Model file for the job. Use its own axes, mm. Face numbers are marked on the shaded views. A direction names the side the tool comes from. Coordinates: 2 decimals unless noted, no trailing zeros. Order: outer loops, then holes, each group sorted by start corner. A loop starts at its lowest first (then second) coordinate and runs counter-clockwise, first axis right, second up. Notation, with made-up numbers: M 38.25,51.25 L 43.25,51.25 A18 cw 43.25,64.25 Z; hole C 81,-14.75 d7. An arc over 180 degrees is marked long. Return JSON: item names as keys, results as strings.
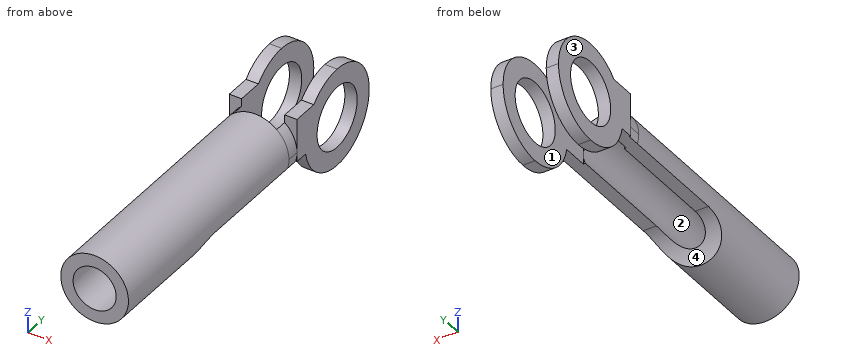
```python
from build123d import *
from build123d.topology import SkipClean

# Parameters (mm, degrees)
SKETCH_1_R               = 2.75
SKETCH_1_R_2             = 1.75
EXTRUDE_1_DEPTH          = 20
CUT_EXTRUDE_2_DEPTH      = 21.374616561
CUT_EXTRUDE_2_DEPTH_BACK = 21.374616561
SKETCH_3_W               = 1
SKETCH_3_H               = 8
EXTRUDE_3_DEPTH          = 10
SKETCH_4_R               = 2.5
CUT_EXTRUDE_5_DEPTH      = 31.761176848
CUT_EXTRUDE_8_DEPTH      = 1


with BuildPart() as part:
    # 草圖1 → 伸長1 (new body)
    with BuildSketch(Plane(origin=(0, 0, 0), x_dir=(1, 0, 0), z_dir=(0, 1, 0))):
        with Locations(Location((0, 0, 0), (0, 0, 270))):
            Circle(SKETCH_1_R)
        with Locations(Location((0, 0, 0), (0, 0, 270))):
            Circle(SKETCH_1_R_2, mode=Mode.SUBTRACT)
    extrude(amount=EXTRUDE_1_DEPTH)

    # 草圖2 → 伸長2 (cut, two sides: drawn at the far end of the back side and taken through both)
    with BuildSketch(Plane(origin=(0, 0, 0), x_dir=(0, 0, -1), z_dir=(1, 0, 0)).offset(-CUT_EXTRUDE_2_DEPTH_BACK)):
        with BuildLine():
            Line((0.75, 20), (0.75, 11.16227766))
            ThreePointArc((0.75, 11.16227766), (1.291960108, 9.291448967), (2.75, 8))
            Line((2.75, 8), (2.75, 20))
            Line((2.75, 20), (0.75, 20))
        make_face()
    extrude(amount=CUT_EXTRUDE_2_DEPTH + CUT_EXTRUDE_2_DEPTH_BACK, mode=Mode.SUBTRACT)

    # 草圖3 → 伸長3 (add)
    with BuildSketch(Plane(origin=(0, 20, 0), x_dir=(1, 0, 0), z_dir=(0, 1, 0))):
        with Locations((-2.25, 0)):
            Rectangle(SKETCH_3_W, SKETCH_3_H)
        with Locations((2.25, 0)):
            Rectangle(SKETCH_3_W, SKETCH_3_H)
    extrude(amount=EXTRUDE_3_DEPTH)

    # 草圖4 → 伸長5 (cut, through all)
    with BuildSketch(Plane.ZY.offset(2.75)):
        with BuildLine():
            Line((-4, 20), (-0.75, 20))
            Line((-0.75, 20), (-0.75, 22.070941589))
            ThreePointArc((-0.75, 22.070941589), (-3.082207, 23.450490242), (-4, 25.999999996))
            Line((-4, 25.999999996), (-4, 20))
        make_face()
        with BuildLine():
            Line((4, 20), (4, 26))
            ThreePointArc((4, 26), (3.674234614, 24.41886117), (2.75, 23.09526249))
            Line((2.75, 23.09526249), (2.75, 20))
            Line((2.75, 20), (4, 20))
        make_face()
        with BuildLine():
            Line((4, 30), (0, 30))
            ThreePointArc((0, 30), (2.828427125, 28.828427125), (4, 26))
            Line((4, 26), (4, 30))
        make_face()
        with BuildLine():
            Line((-4, 30), (-4, 25.999999996))
            ThreePointArc((-4, 25.999999996), (-2.828427126, 28.828427123), (0, 30))
            Line((0, 30), (-4, 30))
        make_face()
        with Locations((0, 26)):
            Circle(SKETCH_4_R)
    extrude(amount=-CUT_EXTRUDE_5_DEPTH, mode=Mode.SUBTRACT)

    # 草圖10 → 伸長8 (cut)
    with SkipClean():  # the faces are left unmerged after this step: merging them gives an invalid solid
        with BuildSketch(Plane.XZ.offset(-20)):
            with BuildLine():
                Line((0, 2.75), (-2.75, 2.75))
                Line((-2.75, 2.75), (-2.75, 0))
                ThreePointArc((-2.75, 0), (-1.944543648, 1.944543648), (0, 2.75))
            make_face()
            with BuildLine():
                Line((2.75, 0), (2.75, 2.75))
                Line((2.75, 2.75), (1.75, 2.75))
                Line((1.75, 2.75), (1.75, 2.121320344))
                ThreePointArc((1.75, 2.121320344), (2.487468593, 1.17260394), (2.75, 0))
            make_face()
            with BuildLine():
                Line((1.75, 2.75), (0, 2.75))
                ThreePointArc((0, 2.75), (0.929749712, 2.588062108), (1.75, 2.121320344))
                Line((1.75, 2.121320344), (1.75, 2.75))
            make_face()
            with BuildLine():
                ThreePointArc((-2.645751311, -0.75), (-2.723813146, -0.378605266), (-2.75, 0))
                Line((-2.75, 0), (-2.75, -0.75))
                Line((-2.75, -0.75), (-2.645751311, -0.75))
            make_face()
            with BuildLine():
                Line((2.75, -0.75), (2.75, 0))
                ThreePointArc((2.75, 0), (2.723813146, -0.378605266), (2.645751311, -0.75))
                Line((2.645751311, -0.75), (2.75, -0.75))
            make_face()
        extrude(amount=-CUT_EXTRUDE_8_DEPTH, mode=Mode.SUBTRACT)


solid = part.part
```
Item 1: Saw through at D-D (y = 13). Write the cut outline in (x, z), and give its area (3 significant figures).
Check result:
{"outline": "M -2.65,-0.75 L -1.58,-0.75 A1.75 cw long 1.58,-0.75 L 2.65,-0.75 A2.75 ccw long Z", "area": "8.60 mm2"}
Item 2: Saw through at C-C (x = 2.15). Write the cut outline in (y, z), and give its area (3 significant figures).
Check result:
{"outline": "M 0,-1.71 L 8.75,-1.71 A3.5 cw 11.16,-0.75 L 22.07,-0.75 A4 ccw long 23.1,2.75 L 21,2.75 L 21,1.71 L 0,1.71 Z; hole C 26,0 d5", "area": "96.0 mm2"}
Item 3: 3-axis set-ups, long thin cutter, end or side, ignore diameter. For the marked faces 1 and 2: which of +Z, -Z, +X, -X, +Y, -Y reach the whole face in a straight line?
Check result:
{"face 1": "+Z, -Z, +Y", "face 2": "+Y, -Y"}
Item 4: Drop flat-ended pins along their axis: pin 1 Ø2 at (y, z) = (15.5, 2.5) entering from +X; pin 2 Ø1.1 at (x, y) = (-2, 22) entering from +Z; pin 3 Ø1.5 at (x, y) = (1.5, 6.5) entering from -Z. Give the stop position or say it passes through.
Check result:
{"pin 1": "stops at x = 2.3", "pin 2": "stops at z = 2.75", "pin 3": "stops at z = -2.65"}
Item 5: Saw through at B-B (y = 3.5). Write the cut outline in (x, z).
Check result:
{"outline": "C 0,0 d5.5; hole C 0,0 d3.5"}
Item 6: Saw through at A-A (x = -0.55). Write the cut outline in (y, z).
Check result:
{"outline": "M 0,-2.69 L 8.03,-2.69 A3.5 cw 8.81,-1.66 L 0,-1.66 Z; M 0,1.66 L 20,1.66 L 20,2.69 L 0,2.69 Z"}
Item 7: Pull direction Y, two halves, no side cores. Call the marked faces 3 and 4: +Y half, -Y half, draft (parallel to the pull), parting line (faces both ways), or undercut.
Check result:
{"face 3": "draft", "face 4": "undercut"}
Item 8: Wall check: line 1 (Y direction, x = -2, z = 0); line 2 (Z direction, x = 0, y = 6.5). Give the ranges that are in metal, low to high.
Check result:
{"line 1": "y = 0 to 23.5, 28.5 to 30", "line 2": "z = -2.75 to -1.75, 1.75 to 2.75"}
